Answer from the drawing. Dimensions are ordinates in mm from the lowest x, y and z of the part. Give positions to 0.01 mm unless a question says otherwise; leave off trailing zeros. Write each loop counter-clockwise with the first axis right and the second up, starting at its lowest first coordinate (ties: lowest second). Pieces come first, ordered by that corner, then holes.
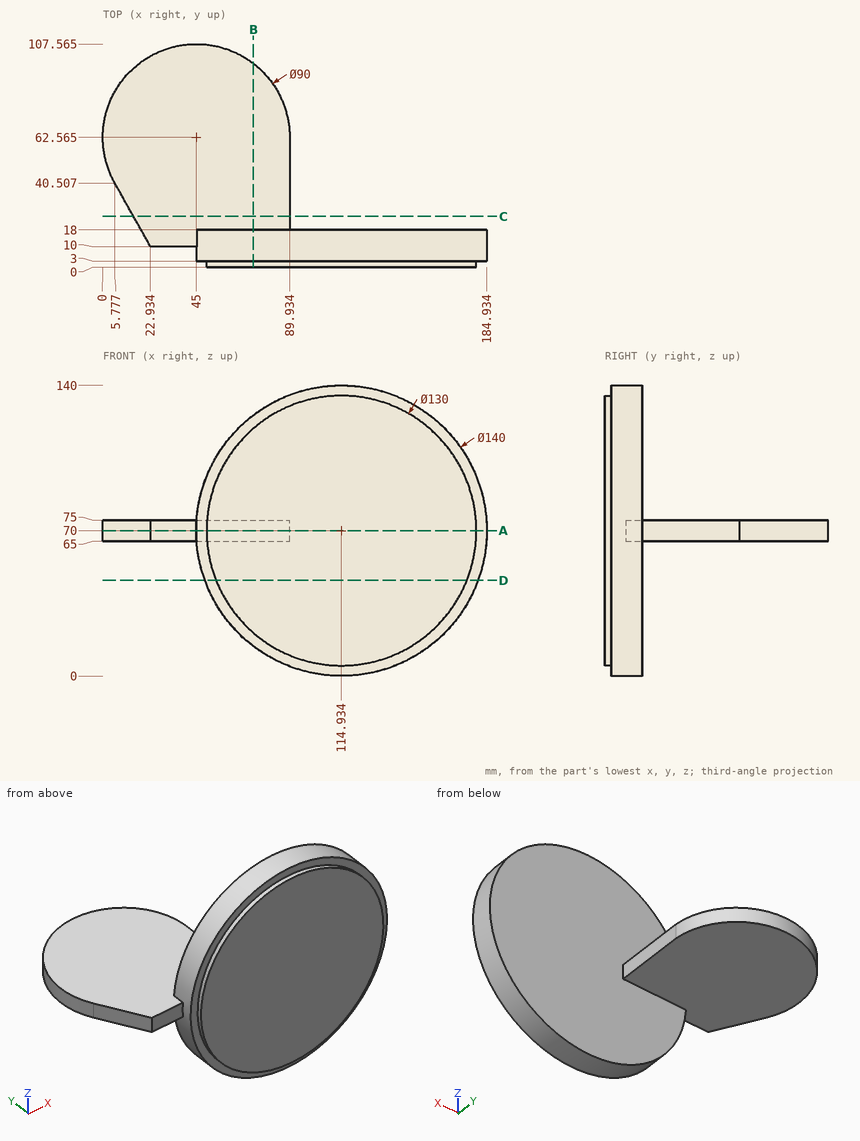
Item 1: A cutting plane is placed at C-C, the plane y = 24.5. Give the vertices of the cut face in (x, z) (1 decimal).
Conclusion:
outline: (14.8, 65) - (89.9, 65) - (89.9, 75) - (14.8, 75) - close
Item 2: Consider probe 1 along Z at (x, y) = (26.5, 25.5); probe 2 along Y at (x, z) = (61, 38); probe 3 along X at (y, z) = (9.5, 69.5) (1 decimal). Determine where each line is inside the solid, lowest interval first.
Conclusion:
probe 1: z = 65 to 75
probe 2: y = 0 to 18
probe 3: x = 44.9 to 184.9
Item 3: A cutting plane is placed at B-B, the plane x = 72.5. Give the vertices of the cut face in (y, z) (1 decimal).
Conclusion:
outline: (0, 20.8) - (3, 20.8) - (3, 14.3) - (18, 14.3) - (18, 65) - (98.2, 65) - (98.2, 75) - (18, 75) - (18, 125.7) - (3, 125.7) - (3, 119.2) - (0, 119.2) - close
Item 4: A cutting plane is placed at D-D, the plane z = 46. Give the vertices of the cut face in (x, y).
Conclusion:
outline: (49.18, 3) - (54.53, 3) - (54.53, 0) - (175.34, 0) - (175.34, 3) - (180.69, 3) - (180.69, 18) - (49.18, 18) - close
Item 5: Each of these flat-tipped pins is pushed along its axis until it touches: P1, Ø6, axis at x = 79, y = 39.5, coming from the +Z side; P2, Ø6, axis at y = 85, z = 75, coming from the -X side; P3, Ø5, axis at x = 39, z = 68, coming from the -Y side. Where does it stop, or does it pass through?
Conclusion:
P1: stops at z = 75
P2: stops at x = 4.41
P3: stops at y = 10
Item 6: A cutting plane is placed at A-A, the plane z = 70. Give the vertices of the cut face in (x, y) (1 decimal).
Conclusion:
outline: (5.8, 40.5) - (22.9, 10) - (44.9, 10) - (44.9, 3) - (49.9, 3) - (49.9, 0) - (179.9, 0) - (179.9, 3) - (184.9, 3) - (184.9, 18) - (89.9, 18) - (89.9, 65) arc R45 ccw (long way) to start
